Read the model definition and answer for the solid it produces. Units are mm, in the model's axes. A direction names the side the tool comes from. Coordinates: 2 decimals unless noted, no trailing zeros. Write each loop counter-clockwise with the first axis right and the second up, starting at its lowest first coordinate (ties: lowest second). Pieces come first, ordered by that corner, then holes.
from build123d import *

# Parameters (mm, degrees)
SKETCH_1_R               = 15
SKETCH_1_R_2             = 1.3
SKETCH_1_W               = 11
SKETCH_1_H               = 5
EXTRUDE_1_DEPTH          = 6
SKETCH_2_W               = 28.284271248
SKETCH_2_H               = 5
EXTRUDE_2_DEPTH          = 30
CUT_EXTRUDE_1_DEPTH      = 44.829214002
CUT_EXTRUDE_1_DEPTH_BACK = 44.829214002
SKETCH_3_R               = 1.5
FILLET_2_R               = 14
SKETCH_4_R               = 2.35
CUT_EXTRUDE_2_DEPTH      = 37.742346223
SKETCH_5_R               = 2.85
CUT_EXTRUDE_3_DEPTH      = 42.785164903
SKETCH_6_R               = 0.75
CUT_EXTRUDE_4_DEPTH      = 1


with BuildPart() as part:
    # 草图1 → 凸台-拉伸1 (new body)
    with BuildSketch(Plane(origin=(0, 0, 0), x_dir=(1, 0, 0), z_dir=(0, 1, 0))):
        with Locations(Location((0, 0, 0), (0, 0, 270))):
            Circle(SKETCH_1_R)
        with Locations(Location((0, 9, 0), (0, 0, 270))):
            Circle(SKETCH_1_R_2, mode=Mode.SUBTRACT)
        with Locations(Location((7.794228634, -4.5, 0), (0, 0, 270))):
            Circle(SKETCH_1_R_2, mode=Mode.SUBTRACT)
        with Locations(Location((-7.794228634, -4.5, 0), (0, 0, 270))):
            Circle(SKETCH_1_R_2, mode=Mode.SUBTRACT)
        with Locations((0, -9.5)):
            Rectangle(SKETCH_1_W, SKETCH_1_H, mode=Mode.SUBTRACT)
    extrude(amount=EXTRUDE_1_DEPTH)

    # 草图2 → 凸台-拉伸2 (add)
    with BuildSketch(Plane(origin=(0, 6, 0), x_dir=(1, 0, 0), z_dir=(0, 1, 0))):
        with Locations((0, 2.5)):
            Rectangle(SKETCH_2_W, SKETCH_2_H)
    extrude(amount=EXTRUDE_2_DEPTH)

    # 草图3 → 切除-拉伸1 (cut, two sides: drawn at the far end of the back side and taken through both)
    with BuildSketch(Plane(origin=(0, 0, -5), x_dir=(-1, 0, 0), z_dir=(0, 0, -1)).offset(-CUT_EXTRUDE_1_DEPTH_BACK)):
        with Locations((-8.25, 14.5)):
            Circle(SKETCH_3_R)
        with Locations((8.25, 14.5)):
            Circle(SKETCH_3_R)
        with Locations((8.25, 29)):
            Circle(SKETCH_3_R)
        with Locations((-8.25, 29)):
            Circle(SKETCH_3_R)
    extrude(amount=CUT_EXTRUDE_1_DEPTH + CUT_EXTRUDE_1_DEPTH_BACK, mode=Mode.SUBTRACT)

    # 圆角2
    # the kernel refuses this fillet: 14 mm, written as the material it adds along each edge
    with BuildSketch(Plane(origin=(49.142135624, 6, 0), x_dir=(0, 0, 1), z_dir=(-1, 0, 0))) as fillet_2_piece_1_section:
        with BuildLine():
            CenterArc((FILLET_2_R, FILLET_2_R), FILLET_2_R, 180, 90)
            Line((0, FILLET_2_R), (0, 0))
            Line((0, 0), (FILLET_2_R, 0))
        make_face()
    fillet_2_piece_1 = extrude(amount=98.284271247, mode=Mode.PRIVATE)
    fillet_2_piece_1 = fillet_2_piece_1 & Plane(origin=(0, 6.047138864, 0), x_dir=(0, 0, 1), z_dir=(0, -1, 0)) * Cylinder(15, 253, mode=Mode.PRIVATE)
    fillet_2_piece_1 = split(fillet_2_piece_1, bisect_by=Plane(origin=(6.949412774, 6.047138864, 12), z_dir=(0, 0, 1)), keep=Keep.TOP, mode=Mode.PRIVATE)
    add(fillet_2_piece_1)
    with BuildSketch(Plane(origin=(14.142135624, 6, 0), x_dir=(0, 0, 1), z_dir=(-1, 0, 0))) as fillet_2_piece_2_section:
        with BuildLine():
            CenterArc((FILLET_2_R, FILLET_2_R), FILLET_2_R, 180, 90)
            Line((0, FILLET_2_R), (0, 0))
            Line((0, 0), (FILLET_2_R, 0))
        make_face()
    fillet_2_piece_2 = extrude(amount=63.284271247, mode=Mode.PRIVATE)
    fillet_2_piece_2 = fillet_2_piece_2 & Plane(origin=(0, 6.60039406, 0), x_dir=(0, 0, 1), z_dir=(0, -1, 0)) * Cylinder(15, 183, mode=Mode.PRIVATE)
    fillet_2_piece_2 = fillet_2_piece_2 - Plane(origin=(7.794228634, 6.60039406, 4.5), x_dir=(0, 0, 1), z_dir=(0, -1, 0)) * Cylinder(1.3, 183, mode=Mode.PRIVATE)
    fillet_2_piece_2 = split(fillet_2_piece_2, bisect_by=Plane(origin=(5.5, 6.60039406, 8.461968408), z_dir=(1, 0, 0)), keep=Keep.TOP, mode=Mode.PRIVATE)
    fillet_2_piece_2 = fillet_2_piece_2 - Plane(origin=(8.25, 14.5, 8.461968408), x_dir=(-1, 0, 0), z_dir=(0, 0, -1)) * Cylinder(1.5, 183, mode=Mode.PRIVATE)
    add(fillet_2_piece_2)
    with BuildSketch(Plane(origin=(49.142135624, 6, 0), x_dir=(0, 0, 1), z_dir=(-1, 0, 0))) as fillet_2_piece_3_section:
        with BuildLine():
            CenterArc((FILLET_2_R, FILLET_2_R), FILLET_2_R, 180, 90)
            Line((0, FILLET_2_R), (0, 0))
            Line((0, 0), (FILLET_2_R, 0))
        make_face()
    fillet_2_piece_3 = extrude(amount=63.284271247, mode=Mode.PRIVATE)
    fillet_2_piece_3 = fillet_2_piece_3 & Plane(origin=(0, 9.416347891, 0), x_dir=(0, 0, 1), z_dir=(0, -1, 0)) * Cylinder(15, 183, mode=Mode.PRIVATE)
    fillet_2_piece_3 = fillet_2_piece_3 - Plane(origin=(-7.794228634, 9.416347891, 4.5), x_dir=(0, 0, 1), z_dir=(0, -1, 0)) * Cylinder(1.3, 183, mode=Mode.PRIVATE)
    fillet_2_piece_3 = split(fillet_2_piece_3, bisect_by=Plane(origin=(0, 9.416347891, 7), z_dir=(0, 0, -1)), keep=Keep.TOP, mode=Mode.PRIVATE)
    fillet_2_piece_3 = split(fillet_2_piece_3, bisect_by=Plane(origin=(5.5, 9.416347891, 2.497543019), z_dir=(-1, 0, 0)), keep=Keep.TOP, mode=Mode.PRIVATE)
    fillet_2_piece_3 = fillet_2_piece_3 - Plane(origin=(-8.25, 14.5, 2.497543019), x_dir=(-1, 0, 0), z_dir=(0, 0, -1)) * Cylinder(1.5, 183, mode=Mode.PRIVATE)
    add(fillet_2_piece_3)
    with BuildSketch(Plane(origin=(49.142135624, 6, 0), x_dir=(0, 0, 1), z_dir=(-1, 0, 0))) as fillet_2_piece_4_section:
        with BuildLine():
            CenterArc((FILLET_2_R, FILLET_2_R), FILLET_2_R, 180, 90)
            Line((0, FILLET_2_R), (0, 0))
            Line((0, 0), (FILLET_2_R, 0))
        make_face()
    fillet_2_piece_4 = extrude(amount=98.284271247, mode=Mode.PRIVATE)
    fillet_2_piece_4 = fillet_2_piece_4 & Plane(origin=(0, 6.600394024, 0), x_dir=(0, 0, 1), z_dir=(0, -1, 0)) * Cylinder(15, 253, mode=Mode.PRIVATE)
    fillet_2_piece_4 = split(fillet_2_piece_4, bisect_by=Plane(origin=(-8.900767253, 6.600394024, 7), z_dir=(0, 0, 1)), keep=Keep.TOP, mode=Mode.PRIVATE)
    fillet_2_piece_4 = split(fillet_2_piece_4, bisect_by=Plane(origin=(-5.5, 6.600394024, 8.461968263), z_dir=(-1, 0, 0)), keep=Keep.TOP, mode=Mode.PRIVATE)
    add(fillet_2_piece_4)

    # 草图4 → 切除-拉伸2 (cut, through all)
    with BuildSketch(Plane(origin=(0, 6, 0), x_dir=(1, 0, 0), z_dir=(0, 1, 0))):
        with Locations((0, 9)):
            Circle(SKETCH_4_R)
        with Locations(Location((7.794228634, -4.5, 0), (0, 0, 90))):
            Circle(SKETCH_4_R)
        with Locations(Location((-7.794228634, -4.5, 0), (0, 0, 90))):
            Circle(SKETCH_4_R)
    extrude(amount=CUT_EXTRUDE_2_DEPTH, mode=Mode.SUBTRACT)

    # 草图5 → 切除-拉伸3 (cut, through all)
    with BuildSketch(Plane.XY):
        with Locations(Location((8.25, 14.5, 0), (0, 0, 236.662521272))):
            Circle(SKETCH_5_R)
        with Locations(Location((-8.25, 14.5, 0), (0, 0, 249.9708463))):
            Circle(SKETCH_5_R)
    extrude(amount=CUT_EXTRUDE_3_DEPTH, mode=Mode.SUBTRACT)

    # 草图6 → 切除-拉伸4 (cut)
    with BuildSketch(Plane(origin=(0, 0, -5), x_dir=(-1, 0, 0), z_dir=(0, 0, -1))):
        with Locations((-12.142135624, 34)):
            Circle(SKETCH_6_R)
    extrude(amount=-CUT_EXTRUDE_4_DEPTH, mode=Mode.SUBTRACT)


solid = part.part
Item 1: Given pin 1 (7.5 mm diameter, centred on x = 7.79, z = 4.5, fed in from +Y); pin 2 (5 mm diameter, centred on x = -8.25, y = 14.5, fed in from +Z); pin 3 (1.5 mm diameter, centred on x = -2.5, y = 7, fed in from -Z); pin 4 (2.5 mm diameter, centred on x = -8.25, y = 29, fed in from -Z), each flat-ended and moving along its own axis, determine where each tip first touches the part or whether it passes through.
Item 2: The part is cut by section C-C (y = 14.5). Give the vertices of the cut face in (x, z), and give its area (3 significant figures).
Item 3: The part is cut by section B-B (x = -8.25). Give the vertices of the cut face in (y, z).
Item 4: The part is cut by section D-D (x = 3). Give the vertices of the cut face in (y, z), and give its area (3 significant figures).
Item 5: For faces 4 (the flat face through (0, 6, -11)), 5 (the cylindrical face through (-8.5, 8.34, 2.26)), 6 (the flat face through (0.1, 6, 14.4)), 7 (the cylindrical face through (-8.377, 11.653, 1.007)), 8 (the flat face through (0, 3, 12)), determine the directions among +Z, -Z, +X, -X, +Y, -Y from which every point of the face is accessible in a straight line to the end or side of a thin tool.
Item 6: Find the intervals of material crossed by probe 1 along X at (y, z) = (7.5, 4.5); probe 2 along X at (y, z) = (14.5, -1.4); probe 3 along Y at (x, z) = (8.25, -2.1), in increasing order.
Item 7: Determine the mould class of faces 1 (the cylindrical face through (0.2, 10.2, 4)), 2 (the cylindrical face through (9.75, 14.57, -2.53)), 3 (the flat face through (-5.5, 3, 10)) for opening direction Z: +Z half, -Z half, draft (parallel to the pull), parting line (faces both ways), or undercut.
Item 8: The part is cut by section A-A (z = -9). Give the vertices of the cut face in (x, y).
Answer:
1. pin 1: stops at y = 13.67
1. pin 2: stops at z = 0
1. pin 3: stops at z = -5
1. pin 4: passes through
2. outline: (-14.14, -5) - (-9.75, -5) - (-9.75, 0) - (-11.1, 0) - (-11.1, 1.13) - (-14.14, 1.13) - close; (-6.75, -5) - (6.75, -5) - (6.75, 0) - (5.4, 0) - (5.4, 1.13) - (-5.4, 1.13) - (-5.4, 0) - (-6.75, 0) - close; (9.75, -5) - (14.14, -5) - (14.14, 1.13) - (11.1, 1.13) - (11.1, 0) - (9.75, 0) - close
2. area: 130 mm2
3. outline: (0, -12.53) - (6, -12.53) - (6, -5) - (13, -5) - (13, 0) - (11.65, 0) - (11.65, 2.19) - (6, 2.19) - (6, 3.28) - (0, 3.28) - close; (0, 5.72) - (6, 5.72) - (6, 6.81) - (7.99, 6.81) arc R14 cw to (6.08, 12.53) - (0, 12.53) - close; (16, -5) - (27.5, -5) - (27.5, 0) - (20, 0) arc R14 cw to (17.35, 0.25) - (17.35, 0) - (16, 0) - close; (30.5, -5) - (36, -5) - (36, 0) - (30.5, 0) - close
4. outline: (0, -14.7) - (6, -14.7) - (6, -5) - (36, -5) - (36, 0) - (20, 0) arc R14 cw to (7.88, 7) - (0, 7) - close; (0, 12) - (6.14, 12) arc R14 cw to (6, 14) - (6, 14.7) - (0, 14.7) - close
4. area: 334 mm2
5. face 4: -Z, +X, -X, +Y
5. face 5: +Y
5. face 6: +Z, +X, -X, +Y
5. face 7: +Z
5. face 8: +Y, -Y
6. probe 1: x = -14.14 to -10.14, -5.44 to 5.44, 10.14 to 14.14
6. probe 2: x = -14.14 to -9.75, -6.75 to 6.75, 9.75 to 14.14
6. probe 3: y = 0 to 13, 16 to 27.5, 30.5 to 36
7. face 1: +Z half
7. face 2: draft
7. face 3: undercut
8. outline: (-12, 0) - (-1.3, 0) - (-1.3, 6) - (-12, 6) - close; (1.3, 0) - (12, 0) - (12, 6) - (1.3, 6) - close
